Part model, mm, in its own coordinate system. A direction names the side the tool comes from. Round coordinates to 2 decimals unless told otherwise and drop trailing zeros. Loops run counter-clockwise (first coordinate to the right, second up) from the corner with the lowest first, then second, coordinate; pieces in that order, holes last. Notation, with made-up numbers: (9, -18) -> (26, -18) arc R18 ccw to (26, -4) -> close; hole circle Ø9 at (62, 41.5). An arc over 180 degrees is marked (long way). Answer as CSV lines item,"result".
from build123d import *

# Parameters (mm, degrees)
SKETCH1_R           = 11
BOSS_EXTRUDE1_DEPTH = 6.35
SKETCH2_R           = 1.9939
CUT_EXTRUDE1_DEPTH  = 7.35
SKETCH14_R          = 1.89865
M3_TAP_DEPTH        = 7.35
SKETCH15_R          = 1.89865
M5_THROUGH_DEPTH    = 7.35
CUT_EXTRUDE2_DEPTH  = 7.35
FILLET2_R           = 6.35


with BuildPart() as part:
    # Sketch1 → Boss-Extrude1 (new body)
    with BuildSketch(Plane(origin=(0, 0, 0), x_dir=(1, 0, 0), z_dir=(0, 1, 0))):
        Polygon((0, 0), (76.2, 0), (76.2, 50.8), (38.1, 50.8), (0, 50.8), align=None)
        with Locations((38.1, 30.8)):
            Circle(SKETCH1_R, mode=Mode.SUBTRACT)
    extrude(amount=BOSS_EXTRUDE1_DEPTH)

    # Sketch2 → Cut-Extrude1 (cut, through all)
    with BuildSketch(Plane(origin=(0, 6.35, 0), x_dir=(1, 0, 0), z_dir=(0, 1, 0))):
        with Locations((19.05, 30.8)):
            Circle(SKETCH2_R)
        with Locations((57.15, 30.8)):
            Circle(SKETCH2_R)
    extrude(amount=-CUT_EXTRUDE1_DEPTH, mode=Mode.SUBTRACT)

    # Sketch14 → M3-tap (cut, through all)
    with BuildSketch(Plane.XZ):
        with Locations((57.15, -44.45)):
            Circle(SKETCH14_R)
        with Locations((19.05, -44.45)):
            Circle(SKETCH14_R)
        with Locations((19.05, -17.15)):
            Circle(SKETCH14_R)
        with Locations((57.15, -17.15)):
            Circle(SKETCH14_R)
    extrude(amount=-M3_TAP_DEPTH, mode=Mode.SUBTRACT)

    # Sketch15 → M5-through (cut, through all)
    with BuildSketch(Plane.XZ):
        with Locations((69.85, -24.45004)):
            Circle(SKETCH15_R)
        with Locations((48.683333333, -6.35)):
            Circle(SKETCH15_R)
        with Locations((27.516666667, -6.35)):
            Circle(SKETCH15_R)
        with Locations((6.35, -24.45004)):
            Circle(SKETCH15_R)
    extrude(amount=-M5_THROUGH_DEPTH, mode=Mode.SUBTRACT)

    # Sketch12 → Cut-Extrude2 (cut, through all)
    with BuildSketch(Plane(origin=(0, 6.35, 0), x_dir=(1, 0, 0), z_dir=(0, 1, 0))):
        Polygon((0, 50.8), (12.7, 50.8), (12.7, 37.15), (0, 24.45), align=None)
        Polygon((63.5, 50.8), (63.5, 37.15), (76.2, 24.45), (76.2, 50.8), align=None)
    extrude(amount=-CUT_EXTRUDE2_DEPTH, mode=Mode.SUBTRACT)

    # Fillet2
    fillet2_edges = [part.edges().sort_by_distance(p)[0] for p in [
        (0, 3.175, -24.45),
        (12.7, 3.175, -50.8),
        (12.7, 3.175, -37.15),
        (63.5, 3.175, -50.8),
        (76.2, 3.175, -24.45),
        (63.5, 3.175, -37.15),
        (76.2, 3.175, 0),
        (0, 3.175, 0),
    ]]
    fillet(fillet2_edges, radius=FILLET2_R)


solid = part.part
Q1. Saw through at B-B, the plane x = 38.1. Write the cut outline in (y, z).
Geometry results:
outline,"(0, -50.8) -> (6.35, -50.8) -> (6.35, -41.8) -> (0, -41.8) -> close; (0, -19.8) -> (6.35, -19.8) -> (6.35, 0) -> (0, 0) -> close"
Q2. Drill centre lines: line 1 along X through (y, z) = (5.25, -30.8); line 2 along Z through (x, y) = (19.05, 2.75); line 3 along Z through (x, y) = (38.5, 2). Where is each one in solid material? Low to high.
Geometry results:
line 1,"6.35 to 17.06, 21.04 to 27.1, 49.1 to 55.16, 59.14 to 69.85"
line 2,"-50.8 to -46.35, -42.55 to -32.79, -28.81 to -19.05, -15.25 to 0"
line 3,"-50.8 to -41.79, -19.81 to 0"
Q3. Drop flat-ended pins along their axis: P1, Ø1, axis at x = 16.5, y = 1.5, coming from the -Z side; P2, Ø2.5, axis at x = 48.68, z = -6.35, coming from the -Y side. Give the stop position or say it passes through.
Geometry results:
P1,"z = -50.46"
P2,"through"
Q4. Two-plate mould, pull along X, no slides. Class faces 4 (the face through (1.91, 3.22, -1.81)), 5 (the face through (38, 3, 0)), 6 (the face through (49.704, 3.131, -4.749)): pulls with the +X half, pulls with the -X half, needs draft (parallel to the pull), parting line crosses it, or undercut.
Geometry results:
face 4,"pulls with the -X half"
face 5,"needs draft"
face 6,"undercut"
Q5. Saw through at D-D, the plane x = 14.5. Write the cut outline in (y, z), then the cut area to 3 significant figures.
Geometry results:
outline,"(0, -48.88) -> (6.35, -48.88) -> (6.35, 0) -> (0, 0) -> close"
area,"310 mm2"
Q6. Saw through at A-A, the plane z = -30.8. Write the cut outline in (x, y), then the cut area to 3 significant figures.
Geometry results:
outline,"(6.35, 0) -> (17.06, 0) -> (17.06, 6.35) -> (6.35, 6.35) -> close; (21.04, 0) -> (27.1, 0) -> (27.1, 6.35) -> (21.04, 6.35) -> close; (49.1, 0) -> (55.16, 0) -> (55.16, 6.35) -> (49.1, 6.35) -> close; (59.14, 0) -> (69.85, 0) -> (69.85, 6.35) -> (59.14, 6.35) -> close"
area,"213 mm2"
Q7. Which spindle directions (+Z, -Z, +X, -X, +Y, -Y) get a long thin tool onto all of the face, cutting with end or side? Do faces 1 (the face through (12.7, 3, -42)), 2 (the face through (63.5, 3, -42)), 3 (the face through (29.328, 3.131, -5.78)). Say none if no direction does.
Geometry results:
face 1,"-Z, -X, +Y, -Y"
face 2,"-Z, +X, +Y, -Y"
face 3,"+Y, -Y"
Q8. Saw through at C-C, the plane y = 3.75. Give the number of separate pieces and of enclosed holes in the cut face, then the cut area to 3 significant figures.
Geometry results:
separate pieces,"1"
enclosed holes,"11"
area,"2,830 mm2"
